Source: three-view drawing plus pictorial views. Frame: mm from the lowest corner of the part. Give positions to 0.01 mm unless a question says otherwise; leave off trailing zeros. Order: outer loops, then holes, each group sorted by start corner. A loop starts at its lowest first (then second) coordinate and runs counter-clockwise, first axis right, second up. Notation, with made-up numbers: (57, 86.25) -> (101, 86.25) arc R32 cw to (101, 116.25) -> close; hole circle Ø6 at (27.5, 58.25). An arc over 180 degrees is marked (long way). One line per question, with ' | ' between items.
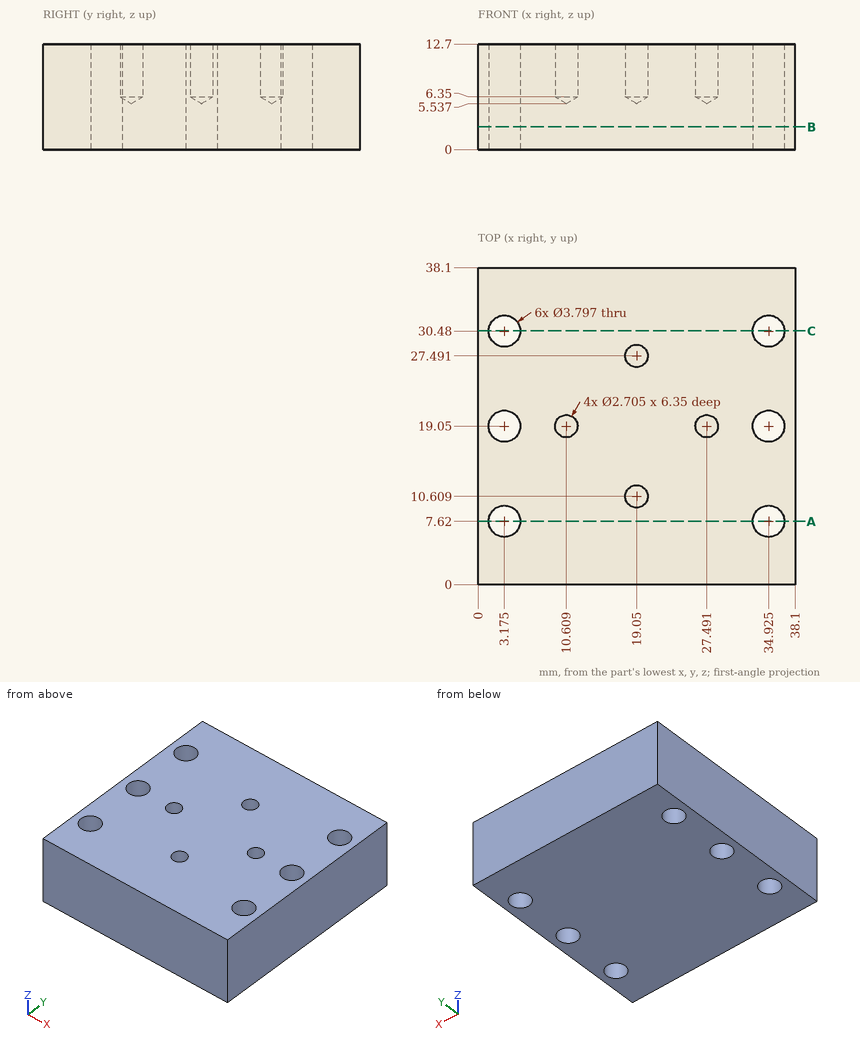
1) Section A-A on y = 7.62. Return loops of the section in (x, z).
Check result:
outline: (0, 0) -> (1.28, 0) -> (1.28, 12.7) -> (0, 12.7) -> close; (5.07, 0) -> (33.03, 0) -> (33.03, 12.7) -> (5.07, 12.7) -> close; (36.82, 0) -> (38.1, 0) -> (38.1, 12.7) -> (36.82, 12.7) -> close
2) Material intervals for probe 1 along X at (y, z) = (7.62, 6); probe 2 along X at (y, z) = (19.05, 10.5); probe 3 along Y at (x, z) = (19, 5.75) (1 decimal), sorted ascending. Write a range as from..to.
Check result:
probe 1: x = 0..1.28, 5.07..33.03, 36.82..38.1 | probe 2: x = 0..1.28, 5.07..9.26, 11.96..26.14, 28.84..33.03, 36.82..38.1 | probe 3: y = 0..10.3, 11..27.1, 27.8..38.1
3) Section B-B on z = 2.75. Count the separate pieces of the cut face and the enclosed holes in it, plus the area to 3 significant figures.
Check result:
separate pieces: 1 | enclosed holes: 6 | area: 1,380 mm^2
4) Contact query for flat-ended pins moving along their axis: pin 1 Ø3.5 at (x, y) = (3.175, 7.62) entering from -Z; pin 2 Ø2 at (x, y) = (19.05, 10.61) entering from +Z. Output: stop coordinate, or through.
Check result:
pin 1: passes through | pin 2: stops at z = 6.14
